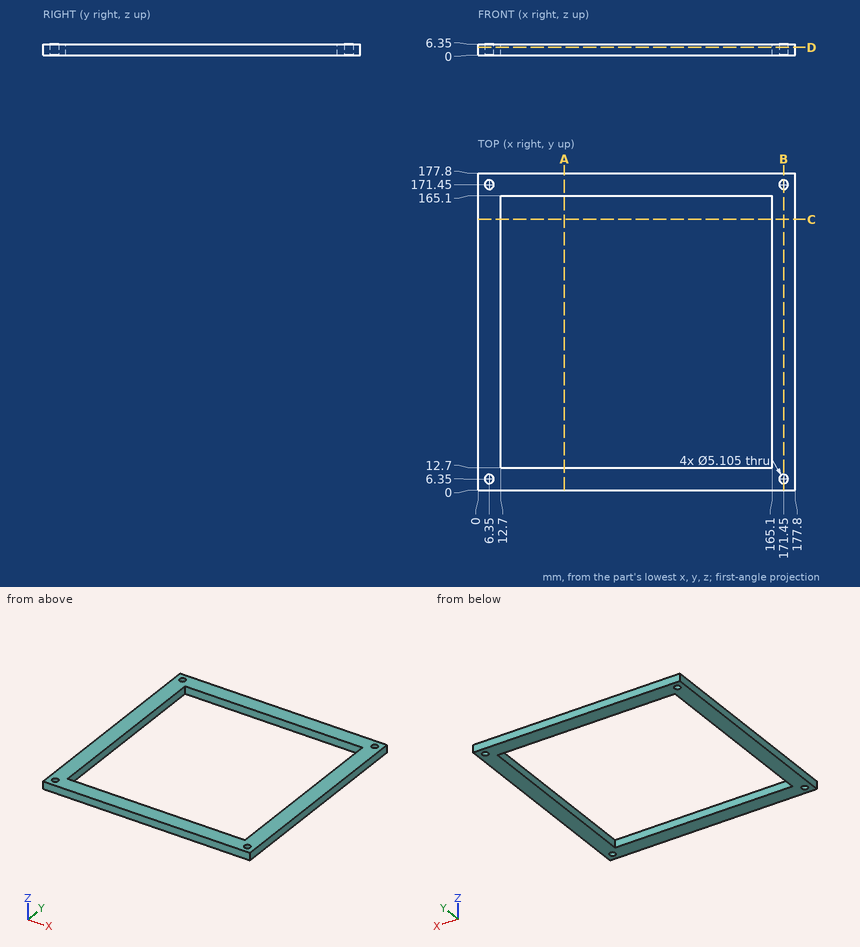
Drawing for the job (mm, zero at the part's lowest x, y, z). Round coordinates to 2 decimals unless told otherwise and drop trailing zeros. Write each loop counter-clockwise with the first axis right and the second up, starting at its lowest first coordinate (ties: lowest second). Pieces come first, ordered by that corner, then holes. Notation, with made-up numbers: M 18,73.5 L 48,73.5 A23 ccw 48,84.5 Z; hole C -5.75,14 d3. An arc over 180 degrees is marked long. Answer as a JSON object with one key per item and string values. Group by question number.
(1) Cut at B-B (x = 171.45). Give the cut face in (y, z), and give its area (3 significant figures).
(2) Drill centre lines: L1, parallel to Y at x = 171.45, z = 2.5; L2, parallel to Y at x = 22, z = 5. Where is each one in solid material? Low to high.
(3) Cut at A-A (x = 48.5). Give the cut face in (y, z).
(4) Cut at D-D (z = 4.5). Give the number of separate pieces and of enclosed holes in the cut face.
Responses:
{
 "1": {"outline": "M 0,0 L 3.8,0 L 3.8,6.35 L 0,6.35 Z; M 8.9,0 L 168.9,0 L 168.9,6.35 L 8.9,6.35 Z; M 174,0 L 177.8,0 L 177.8,6.35 L 174,6.35 Z", "area": "1,060 mm2"},
 "2": {"L1": "y = 0 to 3.8, 8.9 to 168.9, 174 to 177.8", "L2": "y = 0 to 12.7, 165.1 to 177.8"},
 "3": {"outline": "M 0,0 L 12.7,0 L 12.7,6.35 L 0,6.35 Z; M 165.1,0 L 177.8,0 L 177.8,6.35 L 165.1,6.35 Z"},
 "4": {"separate pieces": "1", "enclosed holes": "5"}
}
